```python
from build123d import *

# Parameters (mm, degrees)
Y_KSEKLIK_EKSTR_ZYON1_DEPTH = 7
IZIM2_R                     = 1.5
KES_EKSTR_ZYON1_DEPTH       = 7
PAH1_SIZE                   = 2.5
IZIM3_R                     = 1.75
KES_EKSTR_ZYON2_DEPTH       = 10
KES_EKSTR_ZYON3_START       = -10
IZIM4_R                     = 1.75
KES_EKSTR_ZYON3_DEPTH       = 10
RADYUS1_R                   = 20
IZIM5_W                     = 90
IZIM5_H                     = 10
IZIM5_W_2                   = 10
IZIM5_H_2                   = 66
KES_EKSTR_ZYON4_DEPTH       = 10
RADYUS2_R                   = 4
KES_EKSTR_ZYON5_DEPTH       = 10
IZIM7_R                     = 1.75
KES_EKSTR_ZYON6_DEPTH       = 7
IZIM8_W                     = 10
IZIM8_H                     = 6
KES_EKSTR_ZYON7_DEPTH       = 10
IZIM9_R                     = 1.75
KES_EKSTR_ZYON8_DEPTH       = 10
IZIM10_R                    = 1.75
KES_EKSTR_ZYON9_DEPTH       = 6
KES_EKSTR_ZYON10_START      = -6
IZIM11_R                    = 1.75
KES_EKSTR_ZYON10_DEPTH      = 6
IZIM12_W                    = 4
IZIM12_H                    = 10
KES_EKSTR_ZYON11_DEPTH      = 10


with BuildPart() as part:
    # Çizim1 → Yükseklik-Ekstrüzyon1 (new body)
    with BuildSketch(Plane(origin=(0, 0, 0), x_dir=(1, 0, 0), z_dir=(0, 1, 0))):
        Polygon((0, 0), (0, 53), (15, 53), (30, 66.5), (150, 66.5), (150, -13.5), (30, -13.5), (15, 0), align=None)
    extrude(amount=Y_KSEKLIK_EKSTR_ZYON1_DEPTH)

    # Çizim2 → Kes-Ekstrüzyon1 (cut)
    with BuildSketch(Plane(origin=(0, 7, 0), x_dir=(1, 0, 0), z_dir=(0, 1, 0))):
        with Locations(Location((2.5, 41.25, 0), (0, 0, 270))):
            Circle(IZIM2_R)
        with Locations(Location((2.5, 11.75, 0), (0, 0, 270))):
            Circle(IZIM2_R)
    extrude(amount=-KES_EKSTR_ZYON1_DEPTH, mode=Mode.SUBTRACT)

    # Pah1
    # the kernel refuses this chamfer: 2.5 mm, written as the material it takes off along each edge
    with BuildSketch(Plane(origin=(2.5, 7, -41.25), x_dir=(0, 0, 1), z_dir=(-1, 0, 0))) as pah1_piece_1:
        Polygon((1.5 + PAH1_SIZE, 0), (1.5, -PAH1_SIZE), (1.5, 0), align=None)
    revolve(axis=Axis((2.5, 7, -41.25), (0, 1, 0)), mode=Mode.SUBTRACT)
    with BuildSketch(Plane(origin=(2.5, 7, -11.75), x_dir=(0, 0, 1), z_dir=(-1, 0, 0))) as pah1_piece_2:
        Polygon((1.5 + PAH1_SIZE, 0), (1.5, -PAH1_SIZE), (1.5, 0), align=None)
    revolve(axis=Axis((2.5, 7, -11.75), (0, 1, 0)), mode=Mode.SUBTRACT)

    # Çizim3 → Kes-Ekstrüzyon2 (cut)
    with BuildSketch(Plane.XY.offset(13.5)):
        with Locations((46.24, 3.5)):
            Circle(IZIM3_R)
    extrude(amount=-KES_EKSTR_ZYON2_DEPTH, mode=Mode.SUBTRACT)

    # Çizim4 → Kes-Ekstrüzyon3 (cut)
    with BuildSketch(Plane(origin=(0, 0, -66.5), x_dir=(-1, 0, 0), z_dir=(0, 0, -1)).offset(KES_EKSTR_ZYON3_START)):
        with Locations(Location((-46.24, 3.5, 0), (0, 0, 180))):
            Circle(IZIM4_R)
    extrude(amount=KES_EKSTR_ZYON3_DEPTH, mode=Mode.SUBTRACT)

    # Radyus1
    radyus1_edges = [part.edges().sort_by_distance(p)[0] for p in [
        (150, 3.5, -66.5),
        (150, 3.5, 13.5),
    ]]
    fillet(radyus1_edges, radius=RADYUS1_R)

    # Çizim5 → Kes-Ekstrüzyon4 (cut)
    with BuildSketch(Plane(origin=(0, 7, 0), x_dir=(1, 0, 0), z_dir=(0, 1, 0))):
        with Locations((75, -1.5)):
            Rectangle(IZIM5_W, IZIM5_H)
        with Locations((75, 26.5)):
            Rectangle(IZIM5_W, IZIM5_H)
        with Locations((75, 40.5)):
            Rectangle(IZIM5_W, IZIM5_H)
        with Locations((75, 54.5)):
            Rectangle(IZIM5_W, IZIM5_H)
        with Locations((75, 12.5)):
            Rectangle(IZIM5_W, IZIM5_H)
        with Locations((130, 26.5)):
            Rectangle(IZIM5_W_2, IZIM5_H_2)
    extrude(amount=-KES_EKSTR_ZYON4_DEPTH, mode=Mode.SUBTRACT)

    # Radyus2
    radyus2_edges = [part.edges().sort_by_distance(p)[0] for p in [
        (135, 3.5, -59.5),
        (135, 3.5, 6.5),
    ]]
    fillet(radyus2_edges, radius=RADYUS2_R)

    # Çizim6 → Kes-Ekstrüzyon5 (cut)
    with BuildSketch(Plane(origin=(0, 7, 0), x_dir=(1, 0, 0), z_dir=(0, 1, 0))):
        with BuildLine():
            Line((139, -6), (139, 59))
            ThreePointArc((139, 59), (143.530979443, 53.484870133), (145, 46.5))
            Line((145, 46.5), (145, 6.5))
            ThreePointArc((145, 6.5), (143.530979443, -0.484870133), (139, -6))
        make_face()
    extrude(amount=-KES_EKSTR_ZYON5_DEPTH, mode=Mode.SUBTRACT)

    # Çizim7 → Kes-Ekstrüzyon6 (cut)
    with BuildSketch(Plane(origin=(150, 0, 0), x_dir=(0, 0, -1), z_dir=(1, 0, 0))):
        with Locations((14, 3.5)):
            Circle(IZIM7_R)
        with Locations((39, 3.5)):
            Circle(IZIM7_R)
    extrude(amount=-KES_EKSTR_ZYON6_DEPTH, mode=Mode.SUBTRACT)

    # Çizim8 → Kes-Ekstrüzyon7 (cut)
    with BuildSketch(Plane(origin=(0, 7, 0), x_dir=(1, 0, 0), z_dir=(0, 1, 0))):
        with Locations((5, 26.5)):
            Rectangle(IZIM8_W, IZIM8_H)
    extrude(amount=-KES_EKSTR_ZYON7_DEPTH, mode=Mode.SUBTRACT)

    # Çizim9 → Kes-Ekstrüzyon8 (cut)
    with BuildSketch(Plane(origin=(0, 7, 0), x_dir=(1, 0, 0), z_dir=(0, 1, 0))):
        with Locations(Location((14, 44, 0), (0, 0, 270))):
            Circle(IZIM9_R)
        with Locations(Location((14, 9, 0), (0, 0, 270))):
            Circle(IZIM9_R)
    extrude(amount=-KES_EKSTR_ZYON8_DEPTH, mode=Mode.SUBTRACT)

    # Çizim10 → Kes-Ekstrüzyon9 (cut)
    with BuildSketch(Plane.XY.offset(13.5)):
        with Locations((120.89, 3.5)):
            Circle(IZIM10_R)
    extrude(amount=-KES_EKSTR_ZYON9_DEPTH, mode=Mode.SUBTRACT)

    # Çizim11 → Kes-Ekstrüzyon10 (cut)
    with BuildSketch(Plane(origin=(0, 0, -66.5), x_dir=(-1, 0, 0), z_dir=(0, 0, -1)).offset(KES_EKSTR_ZYON10_START)):
        with Locations(Location((-120.89, 3.5, 0), (0, 0, 180))):
            Circle(IZIM11_R)
    extrude(amount=KES_EKSTR_ZYON10_DEPTH, mode=Mode.SUBTRACT)

    # Çizim12 → Kes-Ekstrüzyon11 (cut)
    with BuildSketch(Plane(origin=(0, 7, 0), x_dir=(1, 0, 0), z_dir=(0, 1, 0))):
        Polygon((26, 56.331873347), (26, 49.5), (22, 49.5), (22, 52.731873347), align=None)
        Polygon((26, -3.5), (22, 0.1), (22, 3.5), (26, 3.5), align=None)
        with Locations((24, 40.5)):
            Rectangle(IZIM12_W, IZIM12_H)
        with Locations((24, 26.5)):
            Rectangle(IZIM12_W, IZIM12_H)
        with Locations((24, 12.5)):
            Rectangle(IZIM12_W, IZIM12_H)
    extrude(amount=-KES_EKSTR_ZYON11_DEPTH, mode=Mode.SUBTRACT)


solid = part.part
```
Input: part model. Units: mm. Frame: model coordinates. A direction names the side the tool comes from. Give positions to 0.01 mm unless a question says otherwise; leave off trailing zeros. Return JSON: item names as keys, results as strings.
1) Contact query for flat-ended pins moving along their axis: pin 1 (3 mm diameter, centred on y = 3.5, z = -14, fed in from +X); pin 2 (2 mm diameter, centred on x = 111.5, z = -10, fed in from -Y). Output: stop coordinate, or through.
Taken from the geometry:
{"pin 1": "stops at x = 139", "pin 2": "passes through"}
2) Mould query, pull axis X, two halves, no side actions, for faces 1 (the face through (5, 4, -23.5)), 2 (the face through (143.986, 3.549, 7.797)), 3 (the face through (122.559, 2.974, -63.458)). Classes: released by +X, released by -X, zero draft, split by the parting line, or undercut.
Taken from the geometry:
{"face 1": "zero draft", "face 2": "released by +X", "face 3": "undercut"}
3) Line query: L1, parallel to X at y = 3.25, z = -34; L2, parallel to Z at x = 34.5, y = 4.5; L3, parallel to X at y = 4.5, z = -55. Output: solid intervals per line, ascending. Write a range as [from, to].
Taken from the geometry:
{"L1": "x = [0, 125], [135, 139], [145, 150]", "L2": "z = [-66.5, -59.5], [-49.5, -45.5], [-35.5, -31.5], [-21.5, -17.5], [-7.5, -3.5], [6.5, 13.5]", "L3": "x = [17.22, 24.52], [26, 30], [120, 125], [135, 139], [142.69, 148.1]"}
4) Section query A-A on x = 46.24. Count the separate pieces of the cut face and the enclosed holes in it, and give its area (3 significant figures).
Taken from the geometry:
{"separate pieces": "8", "enclosed holes": "0", "area": "161 mm2"}
5) Access query for faces 4 (the face through (24, 4, -3.5)), 5 (the face through (59, 0, -18)). Directions: +Z, -Z, +X, -X, +Y, -Y. A direction counts if a zero-diameter tool reaches every point of the face in a straight line with its end or side. Return the directions, or none.
Taken from the geometry:
{"face 4": "+Y, -Y", "face 5": "+Z, -Z, +X, -X, -Y"}
